Design review of the part built by this model. Coordinates are the model's own, in mm. Face numbers are marked on the shaded views. A direction names the side the tool comes from. Give positions to 0.01 mm unless a question says otherwise; leave off trailing zeros. Order: outer loops, then holes, each group sorted by start corner. A loop starts at its lowest first (then second) coordinate and runs counter-clockwise, first axis right, second up. Notation, with made-up numbers: M 58,20 L 72,20 A16 cw 72,45 Z; hole C 31,85 d10. An arc over 180 degrees is marked long. Put each result on its own line as item: value. Start each with the question number.
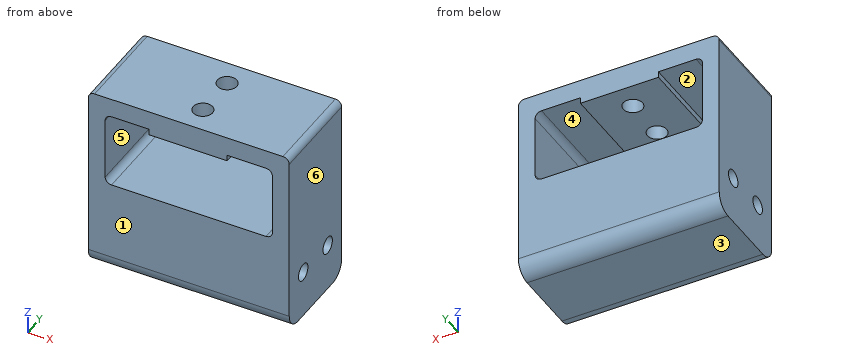
from build123d import *

# Parameters (mm, degrees)
ESQUISSE1_W             = 24.6
ESQUISSE1_H             = 30
BOSS_EXTRU_1_DEPTH      = 1.9
ESQUISSE2_W             = 52.7
ESQUISSE2_H             = 30
BOSS_EXTRU_2_DEPTH      = 6
ESQUISSE4_W             = 29.6
ESQUISSE4_H             = 30
BOSS_EXTRU_3_DEPTH      = 5.3
ESQUISSE5_W             = 29.6
ESQUISSE5_H             = 30
BOSS_EXTRU_4_DEPTH      = 5.3
ESQUISSE6_W             = 63.3
ESQUISSE6_H             = 30
BOSS_EXTRU_5_DEPTH      = 3
CONG_1_R                = 2
ESQUISSE7_W             = 63.3
ESQUISSE7_H             = 30
BOSS_EXTRU_6_DEPTH      = 27
CONG_3_R                = 5
ESQUISSE3_R             = 3.05
ENL_V_MAT_EXTRU_2_DEPTH = 26
ESQUISSE8_R             = 2.7
ENL_V_MAT_EXTRU_3_DEPTH = 68


with BuildPart() as part:
    # Esquisse1 → Boss.-Extru.1 (new body)
    with BuildSketch(Plane.XY):
        with Locations((-0.2, -1.155063291)):
            Rectangle(ESQUISSE1_W, ESQUISSE1_H)
    extrude(amount=BOSS_EXTRU_1_DEPTH)

    # Esquisse2 → Boss.-Extru.2 (add)
    with BuildSketch(Plane.XY.offset(1.9)):
        with Locations((0, -1.155063291)):
            Rectangle(ESQUISSE2_W, ESQUISSE2_H)
    extrude(amount=BOSS_EXTRU_2_DEPTH)

    # Esquisse4 → Boss.-Extru.3 (add)
    with BuildSketch(Plane.ZY.offset(26.35)):
        with Locations((-6.9, -1.155063291)):
            Rectangle(ESQUISSE4_W, ESQUISSE4_H)
    extrude(amount=BOSS_EXTRU_3_DEPTH)

    # Esquisse5 → Boss.-Extru.4 (add)
    with BuildSketch(Plane(origin=(26.35, 0, 0), x_dir=(0, 0, -1), z_dir=(1, 0, 0))):
        with Locations((6.9, -1.155063291)):
            Rectangle(ESQUISSE5_W, ESQUISSE5_H)
    extrude(amount=BOSS_EXTRU_4_DEPTH)

    # Esquisse6 → Boss.-Extru.5 (add)
    with BuildSketch(Plane(origin=(0, 0, -21.7), x_dir=(-1, 0, 0), z_dir=(0, 0, -1))):
        with Locations((0, -1.155063291)):
            Rectangle(ESQUISSE6_W, ESQUISSE6_H)
    extrude(amount=BOSS_EXTRU_5_DEPTH)

    # Congé1
    cong_1_edges = [part.edges().sort_by_distance(p)[0] for p in [
        (-26.35, -1.155063291, 1.9),
        (26.35, -1.155063291, 1.9),
        (-26.35, -1.155063291, -21.7),
        (-31.65, -1.155063291, 7.9),
        (26.35, -1.155063291, -21.7),
        (31.65, -1.155063291, 7.9),
    ]]
    fillet(cong_1_edges, radius=CONG_1_R)

    # Esquisse7 → Boss.-Extru.6 (add)
    with BuildSketch(Plane(origin=(0, 0, -24.7), x_dir=(-1, 0, 0), z_dir=(0, 0, -1))):
        with Locations((0, -1.155063291)):
            Rectangle(ESQUISSE7_W, ESQUISSE7_H)
    extrude(amount=BOSS_EXTRU_6_DEPTH)

    # Congé3
    cong_3_edges = [part.edges().sort_by_distance(p)[0] for p in [
        (0, -16.155063291, -51.7),
        (0, 13.844936709, -51.7),
    ]]
    fillet(cong_3_edges, radius=CONG_3_R)

    # Esquisse3 → Enlèv. mat.-Extru.2 (cut)
    with BuildSketch(Plane.XY):
        with Locations(Location((0, 5.769936709, 0), (0, 0, 180))):
            Circle(ESQUISSE3_R)
        with Locations(Location((0, -8.080063291, 0), (0, 0, 180))):
            Circle(ESQUISSE3_R)
    extrude(amount=ENL_V_MAT_EXTRU_2_DEPTH, mode=Mode.SUBTRACT)

    # Esquisse8 → Enlèv. mat.-Extru.3 (cut)
    with BuildSketch(Plane.ZY.offset(31.65)):
        with Locations(Location((-36.7, 5.844936709, 0), (0, 0, 270))):
            Circle(ESQUISSE8_R)
        with Locations(Location((-36.7, -8.155063291, 0), (0, 0, 270))):
            Circle(ESQUISSE8_R)
    extrude(amount=-ENL_V_MAT_EXTRU_3_DEPTH, mode=Mode.SUBTRACT)


solid = part.part
1. To check wall thickness, follow probe 1 along Z at (x, y) = (10, -8); probe 2 along Y at (x, z) = (0, 6.5); probe 3 along X at (y, z) = (-3.5, -10). State the ranges of each line that lie inside material, in increasing order.
2. Consider section C-C on x = 0. Give the boundary of the cut face in (y, z), then the cut area to 3 significant figures.
3. Insertion check: pin 1 (4 mm diameter, centred on x = 20.5, y = -12.5, fed in from -Z). The pin has a flat end and moves straight along its axis. Give the tip position at first contact, or say it passes through.
4. Machinability: for the marked faces 1 and 2, which of the approach directions +Z, -Z, +X, -X, +Y, -Y give a long, thin tool a straight path to every point of the face, cutting with its end or side? Answer none if there is none.
5. Consider section A-A on x = -10.5. Give the boundary of the cut face in (y, z), then the cut area to 3 significant figures.
6. Consider section D-D on z = -4. Give the boundary of the cut face in (x, y).
7. The part is to be moulded in two halves that separate along X. For the marked faces 3, 4, 5 and 6, say which applies: +X half, -X half, draft (parallel to the pull), parting line (faces both ways), or undercut.
8. Consider section B-B on z = -36.7. Give the boundary of the cut face in (x, y), then the cut area to 3 significant figures.
Returned:
1. probe 1: z = -51.7 to -39.4, -34 to -21.7, 0 to 7.9
1. probe 2: y = -16.16 to -11.13, -5.03 to 2.72, 8.82 to 13.84
1. probe 3: x = -31.65 to -26.35, 26.35 to 31.65
2. outline: M -16.16,-46.7 A5 ccw -11.16,-51.7 L 8.84,-51.7 A5 ccw 13.84,-46.7 L 13.84,-21.7 L -16.16,-21.7 Z; M -16.16,0 L -11.13,0 L -11.13,7.9 L -16.16,7.9 Z; M -5.03,0 L 2.72,0 L 2.72,7.9 L -5.03,7.9 Z; M 8.82,0 L 13.84,0 L 13.84,7.9 L 8.82,7.9 Z; hole C -8.16,-36.7 d5.4; hole C 5.84,-36.7 d5.4
2. area: 984 mm2
3. pin 1: stops at z = -51.7
4. face 1: +Z, -Z, +X, -X, -Y
4. face 2: +Y, -Y
5. outline: M -16.16,-46.7 A5 ccw -11.16,-51.7 L 8.84,-51.7 A5 ccw 13.84,-46.7 L 13.84,-21.7 L -16.16,-21.7 Z; M -16.16,0 L 13.84,0 L 13.84,7.9 L -16.16,7.9 Z; hole C -8.16,-36.7 d5.4; hole C 5.84,-36.7 d5.4
5. area: 1,080 mm2
6. outline: M -31.65,-16.16 L -26.35,-16.16 L -26.35,13.84 L -31.65,13.84 Z; M 26.35,-16.16 L 31.65,-16.16 L 31.65,13.84 L 26.35,13.84 Z
7. face 3: draft
7. face 4: undercut
7. face 5: undercut
7. face 6: +X half
8. outline: M -31.65,-16.16 L 31.65,-16.16 L 31.65,-10.86 L -31.65,-10.86 Z; M -31.65,-5.46 L 31.65,-5.46 L 31.65,3.14 L -31.65,3.14 Z; M -31.65,8.54 L 31.65,8.54 L 31.65,13.84 L -31.65,13.84 Z
8. area: 1,220 mm2
